```python
from build123d import *

# Parameters (mm, degrees)
BOSS_EXTRU_1_DEPTH = 128.5
CONG_1_R           = 6


with BuildPart() as part:
    # Esquisse1 → Boss.-Extru.1 (new body)
    with BuildSketch(Plane.XY):
        with BuildLine():
            Line((-133, -22), (0, -22))
            Line((0, -22), (0, 0))
            Line((0, 0), (-133, 0))
            ThreePointArc((-133, 0), (-190.982756057, -24.017243943), (-215, -82))
            Line((-215, -82), (-215, -424))
            ThreePointArc((-215, -424), (-190.982756057, -481.982756057), (-133, -506))
            Line((-133, -506), (0, -506))
            Line((0, -506), (0, -484))
            Line((0, -484), (-133, -484))
            ThreePointArc((-133, -484), (-175.426406871, -466.426406871), (-193, -424))
            Line((-193, -424), (-193, -82))
            ThreePointArc((-193, -82), (-175.426406871, -39.573593129), (-133, -22))
        make_face()
    extrude(amount=-BOSS_EXTRU_1_DEPTH)

    # Congé1
    cong_1_edges = [part.edges().sort_by_distance(p)[0] for p in [
        (-66.5, 0, -128.5),
        (-190.982756057, -24.017243943, -128.5),
        (-215, -253, -128.5),
        (-190.982756057, -481.982756057, -128.5),
        (-66.5, -506, -128.5),
        (-66.5, -484, -128.5),
        (-175.426406871, -466.426406871, -128.5),
        (-193, -253, -128.5),
        (-175.426406871, -39.573593129, -128.5),
        (-66.5, -22, -128.5),
    ]]
    fillet(cong_1_edges, radius=CONG_1_R)


solid = part.part
```
The model under review builds one solid part; all positions refer to its coordinate system, in mm. A direction names the side the tool comes from. Round coordinates to 2 decimals unless told otherwise and drop trailing zeros. Loops run counter-clockwise (first coordinate to the right, second up) from the corner with the lowest first, then second, coordinate; pieces in that order, holes last. Notation, with made-up numbers: (71.25, -26.75) - (91.25, -26.75) arc R21 cw to (91.25, -22.75) - close; hole circle Ø5 at (-27, -14). An arc over 180 degrees is marked (long way). Write each question's results on one line, items separated by ' | '. Start each with the question number.
Q1. Draft analysis for pull direction Y (two halves, no side actions). For faces 1 (the cylindrical face through (-191.62, -481.34, -60.39)), 2 (the flat face through (-196, -271, 0)), 3 (the flat face through (-67, -22, -60)), state which applies: pulls with the +Y half, pulls with the -Y half, needs draft (parallel to the pull), parting line crosses it, or undercut.
Q2. Take a section at C-C on y = -303. Give the boundary of the cut face in (x, z).
Q3. Insertion check: P1, Ø1, axis at y = -259.5, z = -37, coming from the +X side. The pin has a flat end and moves straight along its axis. Give the tip position at first contact, or say it passes through.
Q4. Take a section at A-A on x = -98. Give the boundary of the cut face in (y, z), plus the area to 3 significant figures.
Q5. Take a section at B-B on z = -37.5. Give the boundary of the cut face in (x, y), plus the area to 3 significant figures.
Q6. Wall thickness on line 1 along Y through (x, z) = (-56, -90); line 2 along X through (y, z) = (-388.5, -100); line 3 along Y through (x, z) = (-144, -44): over which ranges is each line inside the solid? List them lowest first. Write a range as [from, to].
Q7. Tool access review of faces 4 (the cylindrical face through (-175.89, -40.04, -60.39)), 5 (the flat face through (-206, -160, -128.5)): name each direction out of +Z, -Z, +X, -X, +Y, -Y from which nothing blocks a thin tool from reaching the whole face with its end or side.
Data:
1) face 1: pulls with the -Y half | face 2: needs draft | face 3: undercut
2) outline: (-215, -122.5) arc R6 ccw to (-209, -128.5) - (-199, -128.5) arc R6 ccw to (-193, -122.5) - (-193, 0) - (-215, 0) - close
3) P1: stops at x = -193
4) outline: (-506, -122.5) arc R6 ccw to (-500, -128.5) - (-490, -128.5) arc R6 ccw to (-484, -122.5) - (-484, 0) - (-506, 0) - close; (-22, -122.5) arc R6 ccw to (-16, -128.5) - (-6, -128.5) arc R6 ccw to (0, -122.5) - (0, 0) - (-22, 0) - close | area: 5,620 mm²
5) outline: (-215, -424) arc R82 ccw to (-133, -506) - (0, -506) - (0, -484) - (-133, -484) arc R60 cw to (-193, -424) - (-193, -82) arc R60 cw to (-133, -22) - (0, -22) - (0, 0) - (-133, 0) arc R82 ccw to (-215, -82) - close | area: 18,300 mm²
6) line 1: y = [-506, -484], [-22, 0] | line 2: x = [-215, -193] | line 3: y = [-505.26, -482.98], [-23.02, -0.74]
7) face 4: +Z, -Z, +X | face 5: -Z, +X, -X, +Y, -Y
